from build123d import *

# Parameters (mm, degrees)
SKETCH2_R            = 39.5
BOSS_EXTRUDE1_DEPTH  = 1
SKETCH4_R            = 41.25
BOSS_EXTRUDE2_DEPTH  = 1
SKETCH5_R            = 42
BOSS_EXTRUDE3_DEPTH  = 7
SKETCH6_R            = 35
BOSS_EXTRUDE4_DEPTH  = 7
BOSS_EXTRUDE5_DEPTH  = 1
CIRPATTERN1_COUNT    = 10
SKETCH9_R            = 15
BOSS_EXTRUDE6_DEPTH  = 10
SKETCH10_W           = 20
SKETCH10_H           = 42
BOSS_EXTRUDE7_DEPTH  = 42
BOSS_EXTRUDE8_START  = -20
BOSS_EXTRUDE8_DEPTH  = 20
SKETCH12_R           = 15
BOSS_EXTRUDE9_DEPTH  = 10
BOSS_EXTRUDE10_START = 10
SKETCH13_R           = 15
BOSS_EXTRUDE10_DEPTH = 10


with BuildPart() as part:
    # Sketch1 → Revolve1 (revolve)
    with BuildSketch(Plane.XY):
        with BuildLine():
            Line((-35, 0), (0, 0))
            Line((0, 0), (0, -20))
            Line((0, -20), (-40, -20))
            ThreePointArc((-40, -20), (-39.657515479, -9.46062113), (-35, 0))
        make_face()
    revolve(axis=Axis((0, 0, 0), (0, -1, 0)))

    # Sketch2 → Boss-Extrude1 (add)
    with BuildSketch(Plane.XZ.offset(20)):
        Circle(SKETCH2_R)
    extrude(amount=BOSS_EXTRUDE1_DEPTH)

    # Sketch3 → Revolve2 (revolve)
    with BuildSketch(Plane(origin=(0, 0, 0), x_dir=(0, 0, -1), z_dir=(1, 0, 0)), mode=Mode.PRIVATE) as revolve2_sk:
        with BuildLine():
            Line((0, -21), (-40, -21))
            ThreePointArc((-40, -21), (-42.384109041, -30.861589096), (-42, -41))
            Line((-42, -41), (0, -41))
            Line((0, -41), (0, -21))
        make_face()
    revolve(revolve2_sk.sketch.rotate(Axis((0, -21, 0), (0, -1, 0)), 90), axis=Axis((0, -21, 0), (0, -1, 0)))

    # Sketch4 → Boss-Extrude2 (add)
    with BuildSketch(Plane.XZ.offset(41)):
        with Locations(Location((0, 0, 0), (0, 0, 270))):
            Circle(SKETCH4_R)
    extrude(amount=BOSS_EXTRUDE2_DEPTH)

    # Sketch5 → Boss-Extrude3 (add)
    with BuildSketch(Plane.XZ.offset(42)):
        with Locations(Location((0, 0, 0), (0, 0, 270))):
            Circle(SKETCH5_R)
    extrude(amount=BOSS_EXTRUDE3_DEPTH)

    # Sketch6 → Boss-Extrude4 (add)
    with BuildSketch(Plane.XZ.offset(49)):
        with Locations(Location((0, 0, 0), (0, 0, 270))):
            Circle(SKETCH6_R)
    extrude(amount=BOSS_EXTRUDE4_DEPTH)

    # Sketch7 → Boss-Extrude5 (add)
    with BuildSketch(Plane.XZ.offset(49)):
        Polygon((38.446071931, -2.233948034), (40.380727679, -1.116974017), (40.380727679, 1.116974017), (38.446071931, 2.233948034), (36.511416183, 1.116974017), (36.511416183, -1.116974017), align=None)
        Polygon((38.446071931, -1.546904417), (39.785730453, -0.773452208), (39.785730453, 0.773452208), (38.446071931, 1.546904417), (37.106413409, 0.773452208), (37.106413409, -0.773452208), align=None, mode=Mode.SUBTRACT)
    boss_extrude5 = extrude(amount=BOSS_EXTRUDE5_DEPTH)

    # CirPattern1: Boss-Extrude5 ×10 about axis
    cirpattern1_axis = Axis((0, 0, 0), (0, 1, 0))
    for i in range(1, CIRPATTERN1_COUNT):
        add(boss_extrude5.rotate(cirpattern1_axis, i * 360 / CIRPATTERN1_COUNT))

    # Sketch9 → Boss-Extrude6 (add)
    with BuildSketch(Plane.XZ.offset(56)):
        with Locations(Location((0, 0, 0), (0, 0, 270))):
            Circle(SKETCH9_R)
    extrude(amount=BOSS_EXTRUDE6_DEPTH)

    # Sketch10 → Boss-Extrude7 (add)
    with BuildSketch(Plane(origin=(0, 0, 0), x_dir=(1, 0, 0), z_dir=(0, 1, 0))):
        Rectangle(SKETCH10_W, SKETCH10_H)
    extrude(amount=BOSS_EXTRUDE7_DEPTH)

    # Sketch11 → Boss-Extrude8 (add)
    with BuildSketch(Plane(origin=(10, 0, 0), x_dir=(0, 0, -1), z_dir=(1, 0, 0)).offset(BOSS_EXTRUDE8_START)):
        with BuildLine():
            Line((-21, 42), (21, 42))
            ThreePointArc((21, 42), (0, 63), (-21, 42))
        make_face()
    extrude(amount=BOSS_EXTRUDE8_DEPTH)

    # Sketch12 → Boss-Extrude9 (add)
    with BuildSketch(Plane.ZY.offset(10)):
        with Locations(Location((0, 42, 0), (0, 0, 180))):
            Circle(SKETCH12_R)
    extrude(amount=BOSS_EXTRUDE9_DEPTH)

    # Sketch13 → Boss-Extrude10 (add)
    with BuildSketch(Plane(origin=(10, 0, 0), x_dir=(0, 0, -1), z_dir=(1, 0, 0)).offset(BOSS_EXTRUDE10_START)):
        with Locations((0, 42)):
            Circle(SKETCH13_R)
    extrude(amount=-BOSS_EXTRUDE10_DEPTH)


solid = part.part
Check sheet for the modelled part. Datum: model origin and axes. Units: mm. A direction names the side the tool comes from. Coordinates: 2 decimals unless noted, no trailing zeros. Loops run counter-clockwise (first coordinate to the right, second up) from the corner with the lowest first, then second, coordinate; pieces in that order, holes last. Notation, with made-up numbers: (-2, -34.5) -> (27, -34.5) arc R32 ccw to (27, 3.5) -> close; hole circle Ø1 at (-15.5, 47.5). An arc over 180 degrees is marked (long way). Write item = value, one per line. Start each with the question number.
1. Section check B-B on y = 8. Record the cut outline in (x, z), then the cut area to 3 significant figures.
2. Tool access check on faces 4 (the flat face through (-28, -41, 31)), 5 (the flat face through (37, -50, -1)), 6 (the flat face through (-31, -49, 23)). Record the directions out of +Z, -Z, +X, -X, +Y, -Y that give a thin tool (end or side, any length) a straight path to the whole face; none if there is none.
3. Section check C-C on y = -57.5. Record the cut outline in (x, z), then the cut area to 3 significant figures.
4. Material ranges on line 1 (X direction, y = 54, z = 16.5); line 2 (Y direction, x = 17, z = 1); line 3 (Y direction, x = -29, z = -12.5), recorded low to high.
5. Draft check along X on faces 1 (the flat face through (-10, -50, -37)), 2 (the flat face through (31, -49, 23)), 3 (the cylindrical face through (-40.27, -41.49, 8.94)). Enter one of: released by +X, released by -X, zero draft, split by the parting line, or undercut.
6. Section check A-A on y = 47.5. Record the cut outline in (x, z).
7. Depth check by flat-ended pin: P1, Ø0.5, axis at y = -49.5, z = -0.5, coming from the -X side; P2, Ø4, axis at y = -14.5, z = -33.5, coming from the -X side; P3, Ø4.5, axis at x = -37.5, z = 0, coming from the -Y side. Enter the tip coordinate at first touch or a pass-through.
Responses:
q1.outline = (-10, -21) -> (10, -21) -> (10, 21) -> (-10, 21) -> close
q1.area = 840 mm2
q2.face_4 = none
q2.face_5 = +Z, -Z, +X, -Y
q2.face_6 = -Y
q3.outline = circle Ø30 at (0, 0)
q3.area = 707 mm2
q4.line_1 = -10 to 10
q4.line_2 = -56 to 0, 27.03 to 56.97
q4.line_3 = -56 to 0
q5.face_1 = zero draft
q5.face_2 = undercut
q5.face_3 = split by the parting line
q6.outline = (-20, -13.96) -> (-10, -13.96) -> (-10, -20.27) -> (10, -20.27) -> (10, -13.96) -> (20, -13.96) -> (20, 13.96) -> (10, 13.96) -> (10, 20.27) -> (-10, 20.27) -> (-10, 13.96) -> (-20, 13.96) -> close
q7.P1 = -40.38
q7.P2 = -25.27
q7.P3 = -50
